Could you check a few things on this model? Use its own coordinates, in mm. A direction names the side the tool comes from. Round coordinates to 2 decimals unless told otherwise and drop trailing zeros. Write each loop counter-clockwise with the first axis right and the second up, starting at its lowest first coordinate (ties: lowest second). Pieces come first, ordered by that corner, then holes. Notation, with made-up numbers: (9.25, 82.5) -> (25.25, 82.5) arc R20 ccw to (25.25, 116.5) -> close; hole circle Ø4 at (60.5, 82.25). An arc over 180 degrees is marked (long way). Return JSON: item names as keys, results as strings.
from build123d import *

# Parameters (mm, degrees)
BOSS_EXTRUDE1_DEPTH = 1662.1125
SKETCH4_R           = 3.96875
CUT_EXTRUDE3_DEPTH  = 44.45
LPATTERN1_COUNT     = 15
LPATTERN1_PITCH     = 101.6


with BuildPart() as part:
    # Sketch1 → Boss-Extrude1 (new body)
    with BuildSketch(Plane.XY):
        Polygon((0, 0), (-38.1, 0), (-38.1, -3.175), (-3.175, -3.175), (-3.175, -38.1), (0, -38.1), align=None)
    extrude(amount=BOSS_EXTRUDE1_DEPTH)

    # Sketch4 → Cut-Extrude3 (cut)
    with BuildSketch(Plane(origin=(10.670100368, 3.175, 817.757022881), x_dir=(1, 0, 0), z_dir=(0, 1, 0))):
        with Locations((-36.070100368, 697.900772881)):
            Circle(SKETCH4_R)
    cut_extrude3 = extrude(amount=-CUT_EXTRUDE3_DEPTH, mode=Mode.SUBTRACT)

    # LPattern1: Cut-Extrude3 ×15
    with Locations(*[(0, 0, i * LPATTERN1_PITCH) for i in range(1, LPATTERN1_COUNT)]):
        add(cut_extrude3, mode=Mode.SUBTRACT)


solid = part.part
1) I want a section at B-B, the plane z = 297.5. Please give me the cut outline in (x, y) (3 decimals).
Return value:
{"outline": "(-38.1, -3.175) -> (-3.175, -3.175) -> (-3.175, -38.1) -> (0, -38.1) -> (0, 0) -> (-38.1, 0) -> close"}
2) I want a section at A-A, the plane y = -31.5. Please give me the cut outline in (x, z) (1 decimal).
Return value:
{"outline": "(-3.2, 0) -> (0, 0) -> (0, 1662.1) -> (-3.2, 1662.1) -> close"}
3) Will these pins go through, and if not, where does the flat tip stop? pin 1 Ø5 at (x, z) = (-25.4, 1339.06) entering from +Y; pin 2 Ø17.5 at (y, z) = (-16, 1228.5) entering from -X (3 decimals); pin 3 Ø12.5 at (x, z) = (-25.4, 323.06) entering from -Y (3 decimals).
Return value:
{"pin 1": "through", "pin 2": "x = -3.175", "pin 3": "y = -3.175"}
4) For faces 1 (the face through (-21, -3.175, 819)), 2 (the face through (0, -19, 819)), which set-ups out of +Z, -Z, +X, -X, +Y, -Y let a thin tool reach every point of the face, with its end or its side?
Return value:
{"face 1": "+Z, -Z, -X, -Y", "face 2": "+Z, -Z, +X, +Y, -Y"}
5) If I drill on probe 1 along X at (y, z) = (-30, 651) (3 decimals), over which ranges is the centre line in solid material (lowest first)? Write a range as [from, to].
Return value:
{"probe 1": "[-3.175, 0]"}
